from build123d import *

# Parameters (mm, degrees)
SKIZZE1_W                                            = 50
SKIZZE1_H                                            = 40
AUFSATZ_LINEAR_AUSTRAGEN1_DEPTH                      = 5
AUFSATZ_LINEAR_AUSTRAGEN2_DEPTH                      = 3
STIRNSENKUNG_F_R_M3_ZYLINDERSCHRAUBE_MIT_D           = 3.6
STIRNSENKUNG_F_R_M3_ZYLINDERSCHRAUBE_MIT_DEPTH       = 5
STIRNSENKUNG_F_R_M3_ZYLINDERSCHRAUBE_MIT_CBORE_D     = 6.5
STIRNSENKUNG_F_R_M3_ZYLINDERSCHRAUBE_MIT_CBORE_DEPTH = 3.4
SKIZZE6_R                                            = 2
SCHNITT_LINEAR_AUSTRAGEN1_DEPTH                      = 36
SKIZZE7_W                                            = 50
SKIZZE7_H                                            = 3
AUFSATZ_LINEAR_AUSTRAGEN3_DEPTH                      = 12.5


with BuildPart() as part:
    # Skizze1 → Aufsatz-Linear austragen1 (new body)
    with BuildSketch(Plane.XY):
        with Locations((25, -20)):
            Rectangle(SKIZZE1_W, SKIZZE1_H)
    extrude(amount=AUFSATZ_LINEAR_AUSTRAGEN1_DEPTH)

    # Skizze2 → Aufsatz-Linear austragen2 (add)
    with BuildSketch(Plane(origin=(0, 0, 0), x_dir=(1, 0, 0), z_dir=(0, 1, 0))):
        Polygon((25, 30), (16.961524227, 0), (33.038475773, 0), align=None)
    extrude(amount=-AUFSATZ_LINEAR_AUSTRAGEN2_DEPTH)

    # Stirnsenkung für M3 Zylinderschraube mit Innensechskant1
    with Locations(Plane.XY.offset(5)):
        with Locations((15, -10), (35, -10), (35, -30), (15, -30)):
            CounterBoreHole(STIRNSENKUNG_F_R_M3_ZYLINDERSCHRAUBE_MIT_D / 2, STIRNSENKUNG_F_R_M3_ZYLINDERSCHRAUBE_MIT_CBORE_D / 2, STIRNSENKUNG_F_R_M3_ZYLINDERSCHRAUBE_MIT_CBORE_DEPTH, depth=STIRNSENKUNG_F_R_M3_ZYLINDERSCHRAUBE_MIT_DEPTH)

    # Skizze6 → Schnitt-Linear austragen1 (cut, through all)
    with BuildSketch(Plane.XY.offset(5)):
        with Locations((15, -20)):
            Circle(SKIZZE6_R)
        with Locations((35, -20)):
            Circle(SKIZZE6_R)
    extrude(amount=-SCHNITT_LINEAR_AUSTRAGEN1_DEPTH, mode=Mode.SUBTRACT)

    # Skizze7 → Aufsatz-Linear austragen3 (add)
    with BuildSketch(Plane(origin=(0, 0, 0), x_dir=(-1, 0, 0), z_dir=(0, 0, -1))):
        with Locations((-25, -38.5)):
            Rectangle(SKIZZE7_W, SKIZZE7_H)
    extrude(amount=AUFSATZ_LINEAR_AUSTRAGEN3_DEPTH)


solid = part.part
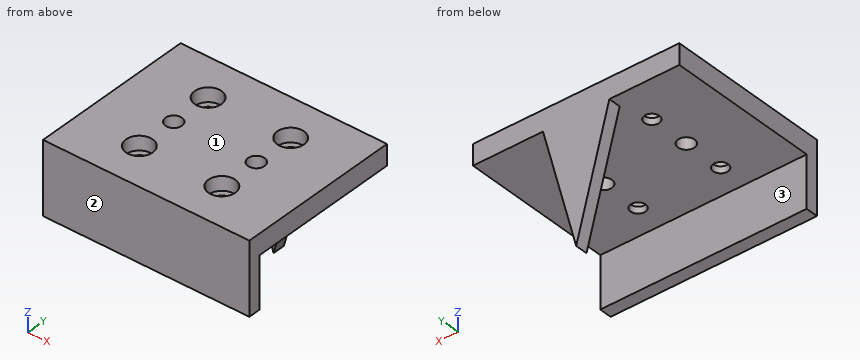
Can you work these out from the model? Positions are in its coordinate system, mm. Face numbers are marked on the shaded views. Coordinates: 2 decimals unless noted, no trailing zeros. Write each loop counter-clockwise with the first axis right and the second up, starting at its lowest first coordinate (ties: lowest second). Pieces come first, ordered by that corner, then holes. Notation, with made-up numbers: M -29.75,7.25 L -14.75,7.25 A6 ccw -14.75,11.25 Z; hole C 28,84.25 d9. An arc over 180 degrees is marked long. Use one line per item in the form item = value.
Q1. I need wall thicknesses on line 1 along Y through (x, z) = (15, 1); line 2 along X through (y, z) = (-10.5, 3.5); line 3 along Y through (x, z) = (21.5, -8). Which ranges of each line are inside material? Lowest first, please. Write a range as from..to.
Model answer:
line_1 = -40..-31.8, -28.2..-22, -18..-11.8, -8.2..0
line_2 = 0..11.79, 18.21..31.79, 38.21..50
line_3 = -40..-37, -3..0
Q2. If we section it at D-D (x = 41.5): Write out the boundary of the cut face in (y, z).
Model answer:
outline = M -40,-12.5 L -37,-12.5 L -37,0 L 0,0 L 0,5 L -40,5 Z
Q3. If we section it at A-A (y = -20): Write out the boundary of the cut face in (x, z).
Model answer:
outline = M 0,0 L 13,0 L 13,5 L 0,5 Z; M 17,0 L 33,0 L 33,5 L 17,5 Z; M 37,0 L 50,0 L 50,5 L 37,5 Z
Q4. If we section it at B-B (x = 15): Write out the boundary of the cut face in (y, z), then the cut area to 3 significant figures.
Model answer:
outline = M -40,-12.5 L -37,-12.5 L -37,0 L -31.8,0 L -31.8,1.6 L -33.25,1.6 L -33.25,5 L -40,5 Z; M -28.2,0 L -22,0 L -22,5 L -26.75,5 L -26.75,1.6 L -28.2,1.6 Z; M -18,0 L -11.8,0 L -11.8,1.6 L -13.25,1.6 L -13.25,5 L -18,5 Z; M -8.2,0 L 0,0 L 0,5 L -6.75,5 L -6.75,1.6 L -8.2,1.6 Z
area = 162 mm^2
Q5. If we section it at C-C (z = -5.5): Write out the boundary of the cut face in (x, y), then the cut area to 3 significant figures.
Model answer:
outline = M 0,-40 L 50,-40 L 50,-37 L 0,-37 Z; M 18.44,-3 L 31.56,-3 L 31.56,0 L 18.44,0 Z
area = 189 mm^2
Q6. We'd pull the mould along Y, two halves only. Please class the marked faces 1, 2 and 3: +Y half, -Y half, draft (parallel to the pull), parting line (faces both ways), or undercut.
Model answer:
face_1 = draft
face_2 = -Y half
face_3 = undercut
Q7. For P1, Ø5, axis at x = 35.5, y = -30, coming from the +Z side; P2, Ø8, axis at x = 11.5, y = -19.5, coming from the -Z side; P3, Ø3, axis at x = 15, y = -10, coming from the -Z side; P4, Ø1, axis at x = 43.5, z = -1, coming from the +Y side, each with a flat end and sliding along its axis, tell me the tip position at first contact or that it passes through.
Model answer:
P1 = 1.6
P2 = 0
P3 = through
P4 = -37
